Geometry: final body of the model. Coordinates: model frame, mm. Face numbers are marked on the shaded views. A direction names the side the tool comes from. Round coordinates to 2 decimals unless told otherwise and drop trailing zeros. Loops run counter-clockwise (first coordinate to the right, second up) from the corner with the lowest first, then second, coordinate; pieces in that order, holes last. Notation, with made-up numbers: (-30, -9.75) - (-16, -9.75) arc R30 cw to (-16, 25.25) - close; hole circle Ø9 at (60, 38.25). An arc over 180 degrees is marked (long way). Return JSON: item names as keys, results as strings. Group by question number.
1. Material intervals for probe 1 along X at (y, z) = (-18.5, 10.25); probe 2 along Y at (x, z) = (24, 4.5); probe 3 along Z at (x, y) = (-6, -18), sorted ascending.
2. Section A-A on z = 14. Return loops of the section in (x, y).
3. First-contact query: pin 1 Ø3 at (x, y) = (19.5, -11) entering from -Z. Flat tip, straight axial feed; report the tip coordinate or a pass-through.
4. Set-up query: the marked faces 1 and 2. Return all of +Z, -Z, +X, -X, +Y, -Y with unobstructed straight access to the full face (end or side cutting, diameter ignored); none if empty.
5. Section C-C on y = -21. Return loops of the section in (x, z), and give its area (3 significant figures).
6. Draft query along Y for the marked faces 3, 4, 5 and 6. Return one class per face: +Y half, -Y half, draft (parallel to the pull), parting line (faces both ways), or undercut.
7. Section B-B on x = 13.5. Return loops of the section in (y, z).
from build123d import *

# Parameters (mm, degrees)
F0_W     = 56.8971335888
F0_H     = 40.2365922928
F1_DEPTH = 25.4
F2_SIZE  = 5.08
F5_T     = -2.54


# Not quite as in the source:
# - the program builds the solid bodies; features that only make, move or delete a surface that nothing else refers to are left out


with BuildPart() as f1:
    # F0 (on Top) → F1 (new body)
    with BuildSketch(Plane.XY):
        with Locations((12.4524980783, -20.1182961464)):
            Rectangle(F0_W, F0_H)
    extrude(amount=F1_DEPTH)

    # F2
    f2_edges = [f1.edges().sort_by_distance(p)[0] for p in [
        (40.901065, -40.236592, 12.7),
        (40.901065, 0, 12.7),
    ]]
    chamfer(f2_edges, length=F2_SIZE)

    # F5
    f5_openings = [f1.faces().sort_by_distance(p)[0] for p in [
        (12.147464, -20.118296, 0),
    ]]
    offset(amount=F5_T, openings=f5_openings)


solid = f1.part
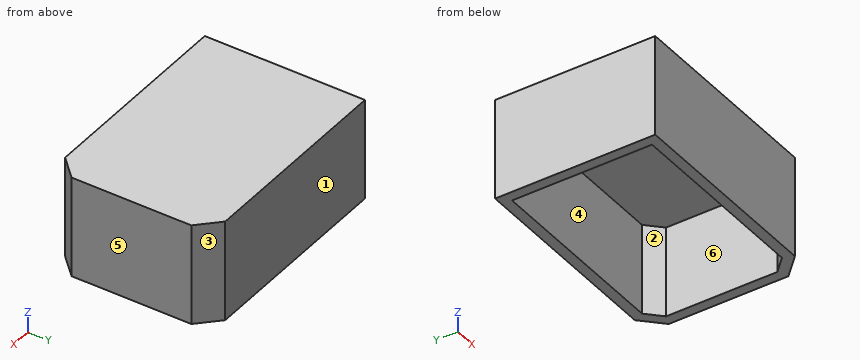
Taken from the geometry:
{
 "1": {"probe 1": "-16 to -13.46, 38.36 to 40.9", "probe 2": "-40.24 to -37.7, -2.54 to 0", "probe 3": "22.86 to 25.4"},
 "2": {"outline": "(-16, -40.24) - (35.82, -40.24) - (40.9, -35.16) - (40.9, -5.08) - (35.82, 0) - (-16, 0) - close; hole (-13.46, -37.7) - (34.77, -37.7) - (38.36, -34.1) - (38.36, -6.13) - (34.77, -2.54) - (-13.46, -2.54) - close"},
 "3": {"pin 1": "z = 22.86"},
 "4": {"face 1": "+Z, -Z, +X, -X, +Y", "face 2": "-Z"},
 "5": {"outline": "(-16, 0) - (-13.46, 0) - (-13.46, 22.86) - (38.36, 22.86) - (38.36, 0) - (40.9, 0) - (40.9, 25.4) - (-16, 25.4) - close", "area": "261 mm2"},
 "6": {"face 3": "+Y half", "face 4": "undercut", "face 5": "draft", "face 6": "undercut"},
 "7": {"outline": "(-40.24, 0) - (-37.7, 0) - (-37.7, 22.86) - (-2.54, 22.86) - (-2.54, 0) - (0, 0) - (0, 25.4) - (-40.24, 25.4) - close"}
}
